The model under review builds one solid part; all positions refer to its coordinate system, in mm. A direction names the side the tool comes from. Round coordinates to 2 decimals unless told otherwise and drop trailing zeros. Order: outer loops, then holes, each group sorted by start corner. A loop starts at its lowest first (then second) coordinate and runs counter-clockwise, first axis right, second up.
Autodesk Inventor part; units mm, degrees
ref_plane "YZ Plane" through (0, 0, 0) normal (1, 0, 0) x (0, 1, 0)
ref_plane "XZ Plane" through (0, 0, 0) normal (0, 1, 0) x (-1, 0, 0)
ref_plane "XY Plane" through (0, 0, 0) normal (0, 0, 1) x (1, 0, 0)
sketch "Esboço1" plane through (0, 0, 0) normal (0, 1, 0) x (-1, 0, 0)
  line L0 (-8, -5) -> (8, -5)
  line L1 (8, -5) -> (8, 5)
  line L2 (8, 5) -> (-8, 5)
  line L3 (-8, 5) -> (-8, -5)
  line L4 (-8, -5) -> (8, 5) construction
  line L5 (8, -5) -> (-8, 5) construction
  point P0 (0, 0)
  dimension "d0" = 16
  dimension "d1" = 10
extrude "Extrusão1" add sketch "Esboço1" along normal blind 4
sketch "Esboço2" plane through (8, 0, 5) normal (1, 0, 0) x (0, 0, -1)
  line L0 (0, 0) -> (0, 4)
  line L1 (10, 0) -> (10, 4)
  line L2 (-0.795, 1.5) -> (-0.795, 2.5)
  line L3 (-0.795, 2.5) -> (6.8544, 2.5)
  line L4 (6.8544, 1.5) -> (-0.795, 1.5)
  line L5 (-0.795, 2.5) -> (8, 2.5)
  line L6 (8.5, 2) -> (8.5, 2)
  line L7 (8, 1.5) -> (-0.795, 1.5)
  line L8 (-0.795, 1.5) -> (-0.795, 2.5)
  arc A0 (8.5, 2) -> (8, 2.5) centre (8, 2) ccw
  arc A1 (8, 1.5) -> (8.5, 2) centre (8, 2) ccw
  point P0 (5, 0)
  point P1 (0, 2.5)
  point P2 (0, 1.5)
  point P3 (8.5, 1.5)
  point P4 (8.5, 2.5)
  dimension "d8" = 1
  dimension "d26" = 9.295
  dimension "d27" = 1
  dimension "d28" = 0.5
chamfer "Chanfro1" distance 1 angle 45 2 edges at (-8, 2, 5) (8, 2, 5)
chamfer "Chanfro2" distance 1 angle 45 2 edges at (0, 4, -5) (0, 0, -5)
chamfer "Chanfro3" distance 0.5 angle 45 4 edges at (8, 4, 0) (8, 0, 0) (-8, 4, 0) (-8, 0, 0)
sketch "Esboço3" plane through (0, 4, 0) normal (0, 1, 0) x (1, 0, 0)
  line L0 (-7.5, -4.5) -> (-7.5, 4)
  line L1 (7, -5) -> (8, -4)
  line L2 (-7.5, 4) -> (7.5, 4)
  line L3 (7.5, 4) -> (7.5, -4.5)
  line L4 (7.5, -4.5) -> (-7.5, -4.5)
  line L5 (-7.5, -4.5) -> (-7.5, 4)
  line L6 (8, 1.8544) -> (-8, 1.8544)
  line L7 (-7.5, 1.8544) -> (7.5, 1.8544)
  line L8 (7.5, 1.8544) -> (7.5, -4.5)
  line L9 (7.5, -4.5) -> (-7.5, -4.5)
  line L10 (-7.5, -4.5) -> (-7.5, 1.8544)
  line L11 (-7.5, -1.3228) -> (7.5, -1.3228)
  line L12 (-7.5, -1.3228) -> (-3.5, -1.3228)
  circle A0 centre (-3.5, -1.3228) radius 1.6
  line L13 (7.5, -1.3228) -> (3.5, -1.3228)
  circle A1 centre (3.5, -1.3228) radius 1.6
  point P0 (0, 0)
  dimension "d20" = 4
  dimension "d21" = 3.2
  dimension "d22" = 4
  dimension "d23" = 3.2
extrude "Extrusão3" cut sketch "Esboço3" against normal through all contours A0 L11 | L11 A0 | A1 L11 | L11 A1
extrude "Extrusão4" cut sketch "Esboço2" against normal through all contours L0 L3 L5 A0 A1 L7 L4
sketch "Esboço4" plane through (8, 1, -5) normal (0, 0, -1) x (-1, 0, 0)
  line L0 (0, 1.5) -> (0, 2.5)
  line L1 (16, 0) -> (16, 2)
  line L2 (16, 2) -> (16, 0)
  line L3 (0, 0) -> (0, 2)
  circle A0 centre (8, 1) radius 1.35
  point P0 (8, -1)
  dimension "d31" = 2.7
sketch "Esboço5" plane through (-7, 0, 5) normal (0, 0, 1) x (1, 0, 0)
  line L0 (0, 4) -> (-0.5, 4)
  line L1 (0, 0) -> (14, 0)
  line L2 (0, 4) -> (14, 4)
  line L3 (14, 4) -> (14, 0)
  line L4 (14, 0) -> (0, 0)
  line L5 (0, 0) -> (0, 4)
  circle A0 centre (7, 2) radius 1.6
  point P0 (7, 0)
  dimension "d32" = 3.2
loft "Transição1" cut profiles "Esboço4", "Esboço5" contours all / A0
properties part number "Sup_haste_corpo"
(1) We need section B-B (z = 1.5). Count the separate pieces of the cut face and the enclosed holes in it, and give its area (3 significant figures).
(2) The part is to be moulded in two halves that separate along X. For faces 4 (the cylindrical face through (3.153, 0.76, 2.885)), 5 (the flat face through (-5.4, 1.5, 0.9)), 6 (the flat face through (8, 1, 0)), say which applies: pulls with the +X half, pulls with the -X half, needs draft (parallel to the pull), parting line crosses it, or undercut.
(3) Tool access review of faces 1 (the flat face through (-7.5, 3.2, 4.5)), 2 (the flat face through (-5.4, 2.5, 1.1)), 3 (the conical face through (0.32, 3.44, 0.07)): name each direction out of +Z, -Z, +X, -X, +Y, -Y from which nothing blocks a thin tool from reaching the whole face with its end or side.
(4) We need section D-D (x = 6.25). Give the boundary of the cut face in (y, z), and give its area (3 significant figures).
(5) We need section A-A (x = -4.25). Give the boundary of the cut face in (y, z).
(6) Clearance check with a flat-ended pin moving along its axis: P1, Ø1.9, axis at x = -3.5, z = 1.32, coming from the -Y side. State where the tip first meets the part, or that it passes through.
(7) To check wall thickness, follow L1, parallel to Y at x = 5.75, z = 1.25; L2, parallel to X at y = 0.35, z = 1.75; L3, parallel to X at y = 0.35, z = 2. State the ranges of each line that lie inside material, in increasing order.
Verdict:
1. separate pieces: 6
1. enclosed holes: 0
1. area: 24.2 mm2
2. face 4: undercut
2. face 5: needs draft
2. face 6: pulls with the +X half
3. face 1: +Z, -X, +Y, -Y
3. face 2: +Z, +X, -X
3. face 3: +Z
4. outline: (0, -4) - (1, -5) - (3, -5) - (4, -4) - (4, 5) - (2.5, 5) - (2.5, -3) arc R0.5 cw to (1.5, -3) - (1.5, 5) - (0, 5) - close
4. area: 30.6 mm2
5. outline: (0, -4) - (1, -5) - (3, -5) - (4, -4) - (4, -0.09) - (2.5, -0.09) - (2.5, -3) arc R0.5 cw to (1.5, -3) - (1.5, -0.09) - (0, -0.09) - close; (0, 2.74) - (1.5, 2.74) - (1.5, 5) - (0, 5) - close; (2.5, 2.74) - (4, 2.74) - (4, 5) - (2.5, 5) - close
6. P1: passes through
7. L1: y = 0 to 1.5, 2.5 to 4
7. L2: x = -7.85 to -5.04, -1.96 to 1.96, 5.04 to 7.85
7. L3: x = -7.85 to -4.95, -2.05 to 2.05, 4.95 to 7.85
